Work out the finished part from the listing and answer in its coordinate system (mm). A direction names the side the tool comes from. Give positions to 0.01 mm unless a question says otherwise; leave off trailing zeros. Order: outer loops, then holes, each group sorted by start corner. A loop starts at its lowest first (then second) coordinate and runs counter-clockwise, first axis right, second up. Notation, with made-up numbers: (-3.5, 84.5) - (42.5, 84.5) arc R16 ccw to (42.5, 97.5) - close; hole circle Ø4 at (75, -5). An arc over 180 degrees is marked (long way). Put each result on its own line as item: value.
```python
from build123d import *

# Parameters (mm, degrees)
F0_W      = 300
F0_H      = 500
F1_DEPTH  = 1850
F2_T      = -2.5
F3_W      = 297.5
F3_H      = 1847.5
F3_W_2    = 277.5
F3_H_2    = 1827.5
F4_DEPTH  = 2.5
F5_R      = 12.5
F6_DEPTH  = 12
F9_DEPTH  = 300.001
F7_R      = 2
F10_DEPTH = 1862.001


with BuildPart() as f1:
    # F0 (on Top) → F1 (new body)
    with BuildSketch(Plane.XY):
        with Locations((150, 250)):
            Rectangle(F0_W, F0_H)
    extrude(amount=F1_DEPTH)

    # F2
    f2_openings = [f1.faces().sort_by_distance(p)[0] for p in [
        (150, 500, 925),
    ]]
    offset(amount=F2_T, openings=f2_openings)

    # F3 (on face) → F4 (join)
    with BuildSketch(Plane(origin=(0, 500, 0), x_dir=(-1, 0, 0), z_dir=(0, 1, 0))):
        with Locations((-148.75, 923.75)):
            Rectangle(F3_W, F3_H)
        with Locations((-148.75, 923.75)):
            Rectangle(F3_W_2, F3_H_2, mode=Mode.SUBTRACT)
    extrude(amount=-F4_DEPTH)

    # F5 (on face) → F6 (join)
    with BuildSketch(Plane(origin=(0, 0, 0), x_dir=(1, 0, 0), z_dir=(0, 0, -1))):
        with Locations((25, -25)):
            Circle(F5_R)
        with Locations((25, -475)):
            Circle(F5_R)
        with Locations((275, -25)):
            Circle(F5_R)
        with Locations((275, -475)):
            Circle(F5_R)
    extrude(amount=F6_DEPTH)

    # F8 (on face) → F9 (cut, through all)
    with BuildSketch(Plane(origin=(0, 0, 0), x_dir=(0, -1, 0), z_dir=(-1, 0, 0))):
        with BuildLine():
            Line((-167, 1730), (-333, 1730))
            ThreePointArc((-333, 1730), (-334.414214, 1729.414214), (-335, 1728))
            Line((-335, 1728), (-335, 1727))
            ThreePointArc((-335, 1727), (-334.414214, 1725.585786), (-333, 1725))
            Line((-333, 1725), (-167, 1725))
            ThreePointArc((-167, 1725), (-165.585786, 1725.585786), (-165, 1727))
            Line((-165, 1727), (-165, 1728))
            ThreePointArc((-165, 1728), (-165.585786, 1729.414214), (-167, 1730))
        make_face()
        with BuildLine():
            ThreePointArc((-335, 1717), (-334.414214, 1715.585786), (-333, 1715))
            Line((-333, 1715), (-167, 1715))
            ThreePointArc((-167, 1715), (-165.585786, 1715.585786), (-165, 1717))
            Line((-165, 1717), (-165, 1718))
            ThreePointArc((-165, 1718), (-165.585786, 1719.414214), (-167, 1720))
            Line((-167, 1720), (-333, 1720))
            ThreePointArc((-333, 1720), (-334.414214, 1719.414214), (-335, 1718))
            Line((-335, 1718), (-335, 1717))
        make_face()
        with BuildLine():
            ThreePointArc((-335, 1707), (-334.414214, 1705.585786), (-333, 1705))
            Line((-333, 1705), (-167, 1705))
            ThreePointArc((-167, 1705), (-165.585786, 1705.585786), (-165, 1707))
            Line((-165, 1707), (-165, 1708))
            ThreePointArc((-165, 1708), (-165.585786, 1709.414214), (-167, 1710))
            Line((-167, 1710), (-333, 1710))
            ThreePointArc((-333, 1710), (-334.414214, 1709.414214), (-335, 1708))
            Line((-335, 1708), (-335, 1707))
        make_face()
        with BuildLine():
            ThreePointArc((-335, 1697), (-334.414214, 1695.585786), (-333, 1695))
            Line((-333, 1695), (-167, 1695))
            ThreePointArc((-167, 1695), (-165.585786, 1695.585786), (-165, 1697))
            Line((-165, 1697), (-165, 1698))
            ThreePointArc((-165, 1698), (-165.585786, 1699.414214), (-167, 1700))
            Line((-167, 1700), (-333, 1700))
            ThreePointArc((-333, 1700), (-334.414214, 1699.414214), (-335, 1698))
            Line((-335, 1698), (-335, 1697))
        make_face()
        with BuildLine():
            ThreePointArc((-335, 1687), (-334.414214, 1685.585786), (-333, 1685))
            Line((-333, 1685), (-167, 1685))
            ThreePointArc((-167, 1685), (-165.585786, 1685.585786), (-165, 1687))
            Line((-165, 1687), (-165, 1688))
            ThreePointArc((-165, 1688), (-165.585786, 1689.414214), (-167, 1690))
            Line((-167, 1690), (-333, 1690))
            ThreePointArc((-333, 1690), (-334.414214, 1689.414214), (-335, 1688))
            Line((-335, 1688), (-335, 1687))
        make_face()
        with BuildLine():
            ThreePointArc((-335, 1677), (-334.414214, 1675.585786), (-333, 1675))
            Line((-333, 1675), (-167, 1675))
            ThreePointArc((-167, 1675), (-165.585786, 1675.585786), (-165, 1677))
            Line((-165, 1677), (-165, 1678))
            ThreePointArc((-165, 1678), (-165.585786, 1679.414214), (-167, 1680))
            Line((-167, 1680), (-333, 1680))
            ThreePointArc((-333, 1680), (-334.414214, 1679.414214), (-335, 1678))
            Line((-335, 1678), (-335, 1677))
        make_face()
    extrude(amount=-F9_DEPTH, mode=Mode.SUBTRACT)

    # F7 (on face) → F10 (cut, through all)
    with BuildSketch(Plane.XY.offset(1850)):
        with Locations((277.5, 495)):
            Circle(F7_R)
    extrude(amount=-F10_DEPTH, mode=Mode.SUBTRACT)


solid = f1.part
```
(1) Determine the mould class of faces 1 (the face through (148, 254, 0)), 2 (the face through (148, 2.5, 912)), 3 (the face through (294, 500, 921)), 4 (the face through (148, 254, 1850)) for opening direction Z: pulls with the +Z half, pulls with the -Z half, needs draft (parallel to the pull), parting line crosses it, or undercut.
Geometry check:
face 1: pulls with the -Z half
face 2: undercut
face 3: needs draft
face 4: pulls with the +Z half
(2) Section A-A, the plane y = 409.5 is taken. Write down the section's boundary in (x, z).
Geometry check:
outline: (0, 0) - (300, 0) - (300, 1850) - (0, 1850) - close; hole (2.5, 2.5) - (297.5, 2.5) - (297.5, 1847.5) - (2.5, 1847.5) - close
(3) Given pin 1 (2 mm diameter, centred on x = 1, y = 271, fed in from -Z); pin 2 (1 mm diameter, centred on x = 50.5, z = 722, fed in from +Y), each flat-ended and moving along its own axis, determine where each tip first touches the part or whether it passes through.
Geometry check:
pin 1: stops at z = 0
pin 2: stops at y = 2.5
(4) Straight lines are drawn through the part: line 1 (Z direction, x = 181, y = 427.5); line 2 (X direction, y = 495, z = 1848.15); line 3 (X direction, y = 202, z = 1298). For each, find the intervals that lie inside material, in ascending order.
Geometry check:
line 1: z = 0 to 2.5, 1847.5 to 1850
line 2: x = 0 to 275.5, 279.5 to 300
line 3: x = 0 to 2.5, 297.5 to 300
(5) Section C-C, the plane x = 243 is taken. Write down the section's boundary in (y, z), then the cut area to 3 significant figures.
Geometry check:
outline: (0, 0) - (500, 0) - (500, 10) - (497.5, 10) - (497.5, 2.5) - (2.5, 2.5) - (2.5, 1847.5) - (497.5, 1847.5) - (497.5, 1837.5) - (500, 1837.5) - (500, 1850) - (0, 1850) - close
area: 7,160 mm²
(6) A tool of negligible diameter and unlimited length cuts with its end or side. For faces 5 (the face through (297.5, 247, 912)), 6 (the face through (148, 0, 912)), from which of +Z, -Z, +X, -X, +Y, -Y can it reach the whole face along a straight path? Write none if from no direction.
Geometry check:
face 5: none
face 6: +Z, -Z, +X, -X, -Y
(7) Section B-B, the plane z = 966 is taken. Write down the section's boundary in (x, y), then the cut area to 3 significant figures.
Geometry check:
outline: (0, 0) - (300, 0) - (300, 500) - (287.5, 500) - (287.5, 497.5) - (297.5, 497.5) - (297.5, 2.5) - (2.5, 2.5) - (2.5, 497.5) - (10, 497.5) - (10, 500) - (0, 500) - close
area: 3,280 mm²
